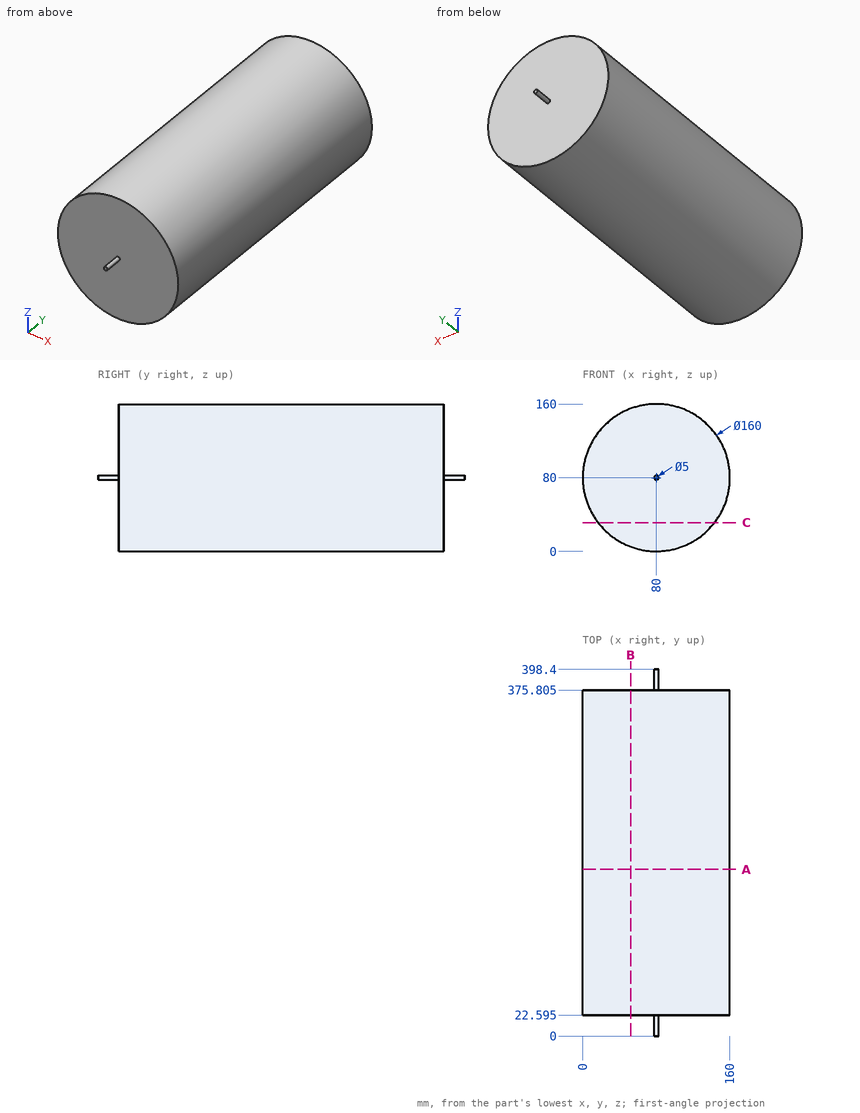
Could you check a few things on this drawing? It's one solid part, dimensions in mm from its lowest x, y, z. Coordinates: 2 decimals unless noted, no trailing zeros. Write each loop counter-clockwise with the first axis right and the second up, starting at its lowest first coordinate (ties: lowest second). Pieces come first, ordered by that corner, then holes. Notation, with made-up numbers: M 16,-4.5 L 72,-4.5 A18 cw 72,29.5 Z; hole C -20.5,-7 d10. An arc over 180 degrees is marked long. One line per question, with ' | ' between items.
1) Imagine slicing it at A-A, the plane y = 181. Write out the boundary of the cut face in (x, z).
Checks:
outline: C 80,80 d160
2) Imagine slicing it at B-B, the plane x = 52. Write out the boundary of the cut face in (y, z) (3 decimals).
Checks:
outline: M 22.595,5.06 L 375.805,5.06 L 375.805,154.94 L 22.595,154.94 Z
3) I need wall thicknesses on probe 1 along Y at (x, z) = (15, 59) (3 decimals); probe 2 along X at (y, z) = (62.5, 81.5); probe 3 along Z at (x, y) = (104.5, 133). Which ranges of each line are inside material? Lowest first, please. Write a range as [from, to].
Checks:
probe 1: [22.595, 375.805] | probe 2: [0.01, 159.99] | probe 3: [3.84, 156.16]
4) Imagine slicing it at C-C, the plane z = 31. Write out the boundary of the cut face in (x, y) (3 decimals), and give its area (3 significant figures).
Checks:
outline: M 16.762,22.595 L 143.238,22.595 L 143.238,375.805 L 16.762,375.805 Z | area: 44,700 mm²
5) For pin 1 Ø5 at (x, y) = (80, 99) entering from +Z; pin 2 Ø3 at (x, z) = (91.5, 49.5) entering from +Y (3 decimals); pin 3 Ø1 at (y, z) = (203.5, 83.5) entering from -X, each with a flat end and sliding along its axis, tell me the tip position at first contact or that it passes through.
Checks:
pin 1: z = 160 | pin 2: y = 375.805 | pin 3: x = 0.06
